Build history of the part. All positions in model axes, mm. A direction names the side the tool comes from. Round coordinates to 2 decimals unless told otherwise and drop trailing zeros. Order: outer loops, then holes, each group sorted by start corner. A loop starts at its lowest first (then second) coordinate and runs counter-clockwise, first axis right, second up. Notation, with made-up numbers: M 33,79 L 45,79 A37 cw 45,116 Z; hole C 43.25,34.25 d9. An arc over 180 degrees is marked long. One line per item, written item: value. Start each with the question number.
Item 1: Pin check, flat tips, straight feed: pin 1 (3 mm diameter, centred on x = 7, y = 6, fed in from +Z); pin 2 (5 mm diameter, centred on x = -10.5, y = 6, fed in from -Z); pin 3 (1.9 mm diameter, centred on x = 3.5, z = -22, fed in from -Y). Stop position of each tip, or through.
Item 2: Band-saw the part on A-A, the plane y = 4.5. Write the cut outline in (x, z).
Item 3: Probe L1, parallel to X at y = 10.5, z = -0.5; L2, parallel to Z at x = -9.5, y = 11.75; L3, parallel to Y at x = 9, z = 1. List the from-to ranges inside material, lowest first.
Item 4: Band-saw the part on B-B, the plane x = -5. Write the cut outline in (y, z).
Item 5: Tool access for faces 1 (the cylindrical face through (21.05, 1.52, -5.13)), 2 (the flat face through (5, 10, 12)), 3 (the flat face through (5, 10, -22)), 4 (the flat face through (5, 8, -15.164)): list every direction of +Z, -Z, +X, -X, +Y, -Y with a clear straight run to the whole face (end or side of a thin tool).
Item 6: Band-saw the part on C-C, the plane z = 3.5. Write the cut outline in (x, y), then the cut area to 3 significant figures.
```python
from build123d import *

# Parameters (mm, degrees)
SKETCH1_W           = 46
SKETCH1_H           = 21
BOSS_EXTRUDE4_DEPTH = 3
SKETCH1_5_W         = 56
SKETCH1_5_H         = 31
SKETCH1_5_W_2       = 46
SKETCH1_5_H_2       = 21
BOSS_EXTRUDE5_DEPTH = 13
BOSS_EXTRUDE6_DEPTH = 3
SKETCH5_R           = 1
CUT_EXTRUDE1_DEPTH  = 1.5
SKETCH6_R           = 1
CUT_EXTRUDE2_DEPTH  = 5


with BuildPart() as part:
    # Sketch1 → Boss-Extrude4 (new body)
    with BuildSketch(Plane(origin=(0, 0, 0), x_dir=(1, 0, 0), z_dir=(0, 1, 0))):
        with Locations((5.163934426, 4.663934426)):
            Rectangle(SKETCH1_W, SKETCH1_H)
    extrude(amount=BOSS_EXTRUDE4_DEPTH)

    # Sketch1_5 → Boss-Extrude5 (add)
    with BuildSketch(Plane(origin=(0, 0, 0), x_dir=(1, 0, 0), z_dir=(0, 1, 0))):
        with Locations((5.163934426, 4.663934426)):
            Rectangle(SKETCH1_5_W, SKETCH1_5_H)
        with Locations((5.163934426, 4.663934426)):
            Rectangle(SKETCH1_5_W_2, SKETCH1_5_H_2, mode=Mode.SUBTRACT)
    extrude(amount=BOSS_EXTRUDE5_DEPTH)

    # Sketch4 → Boss-Extrude6 (add)
    with BuildSketch(Plane(origin=(0, 13, 0), x_dir=(1, 0, 0), z_dir=(0, 1, 0))):
        with BuildLine():
            Line((0.913554246, 20.163934426), (8.664247516, 20.163934426))
            ThreePointArc((8.664247516, 20.163934426), (4.788900881, 24.039281061), (0.913554246, 20.163934426))
        make_face()
        with BuildLine():
            Line((0.913554246, -10.836065574), (8.664247516, -10.836065574))
            ThreePointArc((8.664247516, -10.836065574), (4.788900881, -14.711412209), (0.913554246, -10.836065574))
        make_face()
    extrude(amount=-BOSS_EXTRUDE6_DEPTH)

    # Sketch5 → Cut-Extrude1 (cut)
    with BuildSketch(Plane(origin=(0, 13, 0), x_dir=(1, 0, 0), z_dir=(0, 1, 0))):
        with Locations(Location((4.869123842, 21.345488129, 0), (0, 0, 270))):
            Circle(SKETCH5_R)
        with Locations(Location((4.869123842, -12.017619277, 0), (0, 0, 90))):
            Circle(SKETCH5_R)
    extrude(amount=-CUT_EXTRUDE1_DEPTH, mode=Mode.SUBTRACT)

    # Sketch6 → Cut-Extrude2 (cut)
    with BuildSketch(Plane(origin=(0, 3, 0), x_dir=(1, 0, 0), z_dir=(0, 1, 0))):
        with Locations(Location((-9.836065574, 4.663934426, 0), (0, 0, 270))):
            Circle(SKETCH6_R)
        with Locations(Location((20.163934426, 4.663934426, 0), (0, 0, 90))):
            Circle(SKETCH6_R)
    extrude(amount=-CUT_EXTRUDE2_DEPTH, mode=Mode.SUBTRACT)


solid = part.part
```
Output:
1. pin 1: stops at z = 10.84
1. pin 2: stops at z = -20.16
1. pin 3: stops at y = 10
2. outline: M -22.84,-20.16 L 33.16,-20.16 L 33.16,10.84 L -22.84,10.84 Z; hole M -17.84,-15.16 L 28.16,-15.16 L 28.16,5.84 L -17.84,5.84 Z
3. L1: x = -22.84 to -17.84, 28.16 to 33.16
3. L2: z = -20.16 to -15.16, 5.84 to 10.84
3. L3: y = 0 to 3
4. outline: M 0,-20.16 L 13,-20.16 L 13,-15.16 L 3,-15.16 L 3,5.84 L 13,5.84 L 13,10.84 L 0,10.84 Z
5. face 1: +Y, -Y
5. face 2: +Z, +X, -X, -Y
5. face 3: -Z, +X, -X, -Y
5. face 4: +Y
6. outline: M -22.84,0 L 33.16,0 L 33.16,13 L 28.16,13 L 28.16,3 L -17.84,3 L -17.84,13 L -22.84,13 Z
6. area: 268 mm²
